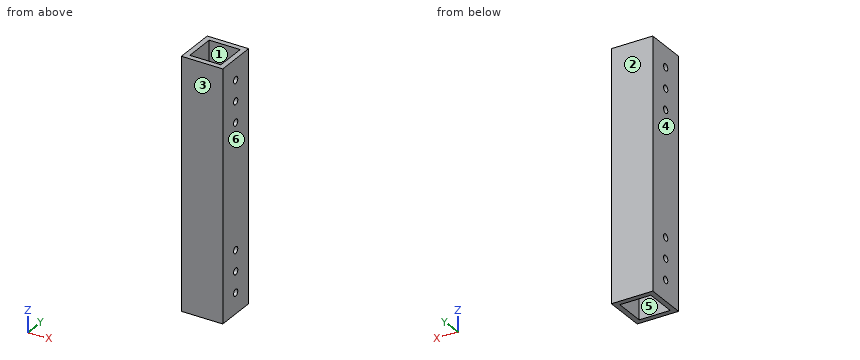
Autodesk Inventor part; units mm, degrees
ref_plane "YZ Plane" through (0, 0, 0) normal (1, 0, 0) x (0, 1, 0)
ref_plane "XZ Plane" through (0, 0, 0) normal (0, 1, 0) x (-1, 0, 0)
ref_plane "XY Plane" through (0, 0, 0) normal (0, 0, 1) x (1, 0, 0)
sketch "Sketch1" plane through (0, 0, 0) normal (0, 0, 1) x (1, 0, 0)
  line L0 (0, 0) -> (25.4, 0)
  line L1 (25.4, 0) -> (25.4, 25.4)
  line L2 (25.4, 25.4) -> (0, 25.4)
  line L3 (0, 25.4) -> (0, 0)
  line L4 (3.175, 22.225) -> (22.225, 22.225)
  line L5 (22.225, 22.225) -> (22.225, 3.175)
  line L6 (22.225, 3.175) -> (3.175, 3.175)
  line L7 (3.175, 3.175) -> (3.175, 22.225)
  dimension "d0" = 25.4
  dimension "d1" = 25.4
  dimension "d3" = 3.175
extrude "Extrusion1" add sketch "Sketch1" along normal blind 152.4
sketch "Sketch2" plane through (25.4, 0, 0) normal (1, 0, 0) x (0, 0, -1)
  line L0 (0, 25.4) -> (-152.4, 25.4)
  line L1 (-152.4, 0) -> (-152.4, 25.4)
  line L2 (0, 0) -> (-152.4, 0)
  circle A0 centre (-139.7, 12.7) radius 2.0701
  circle A1 centre (-127, 12.7) radius 2.0701
  circle A2 centre (-114.3, 12.7) radius 2.0701
  line L3 (-76.2, 25.4) -> (-76.2, 0) construction
  circle A3 centre (-12.7, 12.7) radius 2.0701
  circle A4 centre (-25.4, 12.7) radius 2.0701
  circle A5 centre (-38.1, 12.7) radius 2.0701
  dimension "d6" = 4.1402
  dimension "d7" = 12.7
  dimension "d8" = 12.7
  dimension "d11" = 12.7
extrude "Extrusion2" cut sketch "Sketch2" against normal blind 152.4
properties part number "Clapper Vertical 6 in Segment (4)"
Work out the finished part from the listing and answer in its coordinate system (mm). Face numbers are marked on the shaded views. A direction names the side the tool comes from. Round coordinates to 2 decimals unless told otherwise and drop trailing zeros. Write each loop counter-clockwise with the first axis right and the second up, starting at its lowest first coordinate (ties: lowest second). Pieces come first, ordered by that corner, then holes.
1) A cutting plane is placed at D-D (y = 12.7). Give the number of separate pieces and of enclosed holes in the cut face, plus the area to 3 significant figures.
2) Straight lines are drawn through the part: line 1 (X direction, y = 5.75, z = 22.5) (3 decimals); line 2 (Y direction, x = 1.5, z = 12.7). For each, find the intervals that lie inside material, in ascending order.
3) A tool of negligible diameter and unlimited length cuts with its end or side. For the marked faces 5 and 6, from which of +Z, -Z, +X, -X, +Y, -Y can it reach the whole face along a straight path? Write none if from no direction.
4) A cutting plane is placed at A-A (y = 18.75). Give the vertices of the cut face in (x, z) (3 decimals).
5) A cutting plane is placed at C-C (z = 12.7). Give the vertices of the cut face in (x, y) (3 decimals).
6) The mould has two halves that part along Y. Classify the marked faces 1, 2, 3 and 4: pulls with the +Y half, pulls with the -Y half, needs draft (parallel to the pull), parting line crosses it, or undercut.
Completed:
1. separate pieces: 14
1. enclosed holes: 0
1. area: 810 mm2
2. line 1: x = 0 to 3.175, 22.225 to 25.4
2. line 2: y = 0 to 10.63, 14.77 to 25.4
3. face 5: +Z, -Z
3. face 6: +Z, -Z, +X, +Y, -Y
4. outline: (0, 0) - (3.175, 0) - (3.175, 152.4) - (0, 152.4) - close; (22.225, 0) - (25.4, 0) - (25.4, 152.4) - (22.225, 152.4) - close
5. outline: (0, 0) - (25.4, 0) - (25.4, 10.63) - (22.225, 10.63) - (22.225, 3.175) - (3.175, 3.175) - (3.175, 10.63) - (0, 10.63) - close; (0, 14.77) - (3.175, 14.77) - (3.175, 22.225) - (22.225, 22.225) - (22.225, 14.77) - (25.4, 14.77) - (25.4, 25.4) - (0, 25.4) - close
6. face 1: undercut
6. face 2: pulls with the +Y half
6. face 3: pulls with the -Y half
6. face 4: needs draft
